Can you work these out from the drawing? Everything is in mm from the part's minimum corner. A direction names the side the tool comes from. Give positions to 0.01 mm unless a question says otherwise; leave off trailing zeros. Loops run counter-clockwise (first coordinate to the right, second up) from the corner with the lowest first, then second, coordinate; pieces in that order, holes last. Notation, with made-up numbers: (57.5, -31.75) -> (80.5, -31.75) arc R9 ccw to (80.5, -24.75) -> close; hole circle Ø10 at (84, -15.5). An arc over 180 degrees is marked (long way). Return JSON: item names as keys, results as strings. Group by question number.
Q1. Suppose I cut it at D-D, the plane x = 8. Please give me the cut outline in (y, z), and give its area (3 significant figures).
Q2. I need wall thicknesses on line 1 along Z through (x, y) = (36.65, 38.4); line 2 along X through (y, z) = (38, 36). Which ranges of each line are inside material? Lowest first, please. Write a range as [from, to].
Q3. Suppose I cut it at C-C, the plane y = 52. Please give me the cut outline in (x, z), and give its area (3 significant figures).
Q4. Will these pins go through, and if not, where does the flat tip stop? pin 1 (1.5 mm diameter, centred on x = 36.5, z = 30, fed in from +Y); pin 2 (1.5 mm diameter, centred on x = 36, z = 5.5, fed in from +Y); pin 3 (3.5 mm diameter, centred on x = 20.5, y = 51, fed in from -Z).
Q5. Suppose I cut it at B-B, the plane z = 36.65. Please give me the cut outline in (x, y).
Q6. Which directions (+Z, -Z, +X, -X, +Y, -Y) give clear straight access to the entire face, cutting with the end or side of a thin tool? Please do the marked faces 1 and 2.
Q7. Suppose I cut it at A-A, the plane x = 36.65. Please give me the cut outline in (y, z).
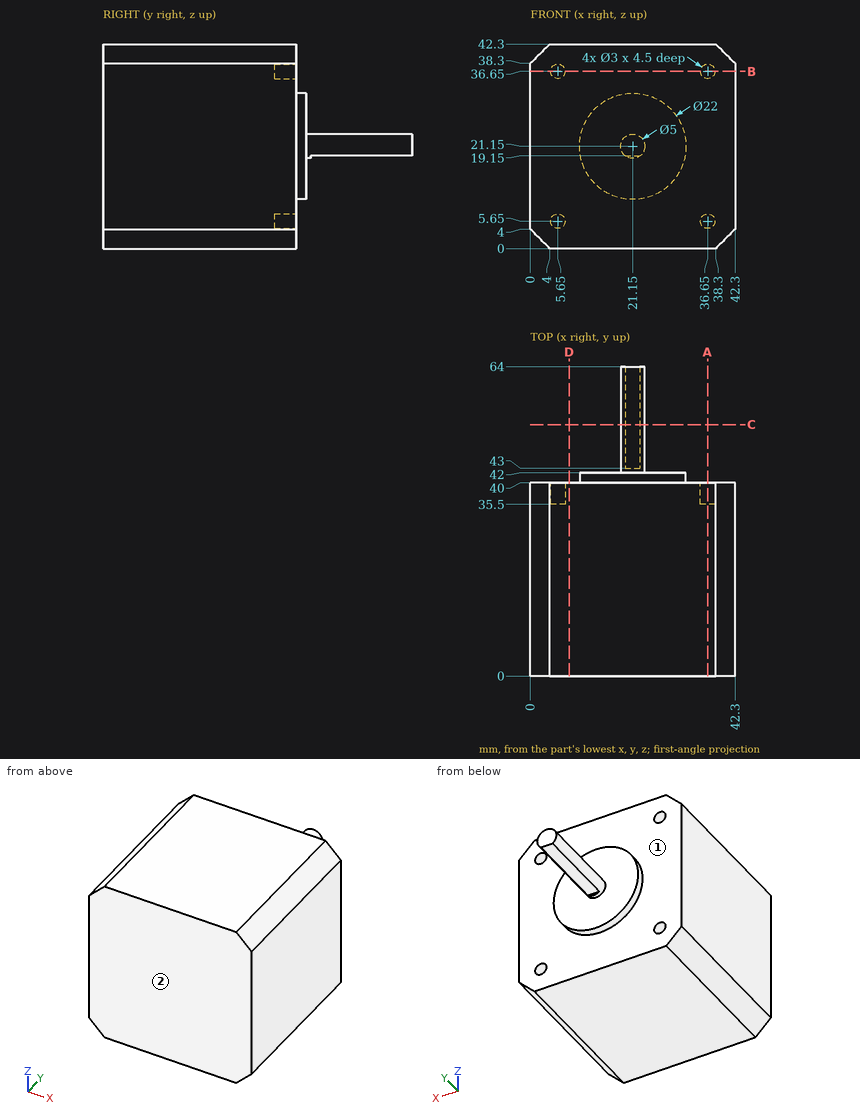
Ans:
{
 "1": {"outline": "(0, 0) -> (40, 0) -> (40, 42.3) -> (0, 42.3) -> close", "area": "1,690 mm^2"},
 "2": {"line 1": "z = [0, 4.15], [7.15, 35.15], [38.15, 42.3]", "line 2": "x = [0, 4.3], [7, 35.3], [38, 42.3]"},
 "3": {"outline": "(19.65, 19.15) -> (22.65, 19.15) arc R2.5 ccw (long way) to start", "area": "18.6 mm^2"},
 "4": {"pin 1": "stops at y = 40", "pin 2": "stops at y = 35.5", "pin 3": "stops at z = 19.15"},
 "5": {"outline": "(0, 0) -> (42.3, 0) -> (42.3, 40) -> (38.15, 40) -> (38.15, 35.5) -> (35.15, 35.5) -> (35.15, 40) -> (7.15, 40) -> (7.15, 35.5) -> (4.15, 35.5) -> (4.15, 40) -> (0, 40) -> close"},
 "6": {"face 1": "+Y", "face 2": "+Z, -Z, +X, -X, -Y"},
 "7": {"outline": "(0, 0) -> (40, 0) -> (40, 4.15) -> (35.5, 4.15) -> (35.5, 7.15) -> (40, 7.15) -> (40, 35.15) -> (35.5, 35.15) -> (35.5, 38.15) -> (40, 38.15) -> (40, 42.3) -> (0, 42.3) -> close"}
}
